Can you work these out from the model? Positions are in its coordinate system, mm. Round coordinates to 2 decimals unless told otherwise and drop trailing zeros. Loops run counter-clockwise (first coordinate to the right, second up) from the corner with the lowest first, then second, coordinate; pieces in that order, holes last.
(1) I want a section at D-D on y = 1.9. Write out the boundary of the cut face in (x, z), plus the area to 3 significant figures.
(2) Will this pin go through, and if not, where does the flat tip stop? pin 1 Ø1.5 at (x, y) = (0, 0) entering from -Z.
(3) I want a section at B-B on z = 0.5. Write out the boundary of the cut face in (x, y), plus the area to 3 significant figures.
(4) I want a section at C-C on x = 1.75. Write out the boundary of the cut face in (y, z), plus the area to 3 significant figures.
(5) I want a section at A-A on x = 0. Write out the boundary of the cut face in (y, z).
(6) If I drill on line 1 along Y through (x, z) = (0, 0.55); line 2 along X through (y, z) = (0.15, 0.1); line 3 along X through (y, z) = (-0.95, -0.1), over which ranges is the centre line in solid material (lowest first)?
(7) Thinking about a two-plate mould opening in Y: for faces 1 (the face through (-0.27, -1.22, -0.01)), 2 (the face through (-2.35, -1.33, 0.01)), 3 (the face through (0, 2.7, 0)), which applies, released by +Y, released by -Y, zero draft, split by the parting line, or undercut?
from build123d import *

# Parameters (mm, degrees)
SKETCH1_R           = 1.25
BOSS_EXTRUDE1_DEPTH = 1
CHAMFER1_SIZE       = 0.3


with BuildPart() as part:
    # Sketch1 → Boss-Extrude1 (new, symmetric)
    with BuildSketch(Plane.XY):
        Polygon((3.117691454, 0), (1.558845727, 2.7), (-1.558845727, 2.7), (-3.117691454, 0), (-1.558845727, -2.7), (1.558845727, -2.7), align=None)
        Circle(SKETCH1_R, mode=Mode.SUBTRACT)
    extrude(amount=BOSS_EXTRUDE1_DEPTH, both=True)

    # Chamfer1
    chamfer1_edges = [part.edges().sort_by_distance(p)[0] for p in [
        (0, 2.7, 1),
        (-2.33826859, 1.35, 1),
        (-2.33826859, -1.35, 1),
        (0, -2.7, 1),
        (2.33826859, -1.35, 1),
        (0, -2.7, -1),
        (-2.33826859, -1.35, -1),
        (-2.33826859, 1.35, -1),
        (0, 2.7, -1),
        (2.33826859, 1.35, -1),
        (2.33826859, -1.35, -1),
        (2.33826859, 1.35, 1),
    ]]
    chamfer(chamfer1_edges, length=CHAMFER1_SIZE)


solid = part.part
Filled sheet:
1. outline: (-2.02, -0.7) - (-1.67, -1) - (1.67, -1) - (2.02, -0.7) - (2.02, 0.7) - (1.67, 1) - (-1.67, 1) - (-2.02, 0.7) - close
1. area: 7.88 mm2
2. pin 1: passes through
3. outline: (-3.12, 0) - (-1.56, -2.7) - (1.56, -2.7) - (3.12, 0) - (1.56, 2.7) - (-1.56, 2.7) - close; hole circle Ø2.5 at (0, 0)
3. area: 20.3 mm2
4. outline: (-2.37, -0.7) - (-1.77, -1) - (1.77, -1) - (2.37, -0.7) - (2.37, 0.7) - (1.77, 1) - (-1.77, 1) - (-2.37, 0.7) - close
4. area: 9.12 mm2
5. outline: (-2.7, -0.7) - (-2.4, -1) - (-1.25, -1) - (-1.25, 1) - (-2.4, 1) - (-2.7, 0.7) - close; (1.25, -1) - (2.4, -1) - (2.7, -0.7) - (2.7, 0.7) - (2.4, 1) - (1.25, 1) - close
6. line 1: y = -2.7 to -1.25, 1.25 to 2.7
6. line 2: x = -3.03 to -1.24, 1.24 to 3.03
6. line 3: x = -2.57 to -0.81, 0.81 to 2.57
7. face 1: undercut
7. face 2: released by -Y
7. face 3: released by +Y
